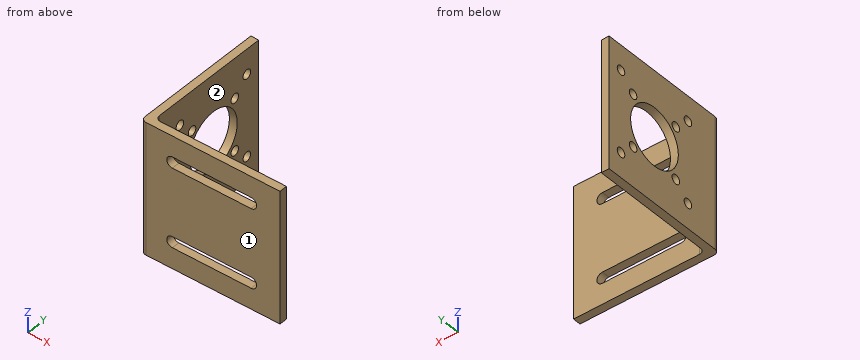
from build123d import *

# Parameters (mm, degrees)
SKETCH1_W           = 53
SKETCH1_H           = 50
BOSS_EXTRUDE1_DEPTH = 3
SKETCH2_W           = 3
SKETCH2_H           = 50
BOSS_EXTRUDE2_DEPTH = 48
CUT_EXTRUDE1_DEPTH  = 4
FILLET1_R           = 2
SKETCH4_R           = 1.75
SKETCH4_R_2         = 11.05
CUT_EXTRUDE2_DEPTH  = 4


with BuildPart() as part:
    # Sketch1 → Boss-Extrude1 (new body)
    with BuildSketch(Plane(origin=(0, 0, 0), x_dir=(1, 0, 0), z_dir=(0, 1, 0))):
        with Locations((26.5, 25)):
            Rectangle(SKETCH1_W, SKETCH1_H)
    extrude(amount=BOSS_EXTRUDE1_DEPTH)

    # Sketch2 → Boss-Extrude2 (add)
    with BuildSketch(Plane(origin=(0, 3, 0), x_dir=(1, 0, 0), z_dir=(0, 1, 0))):
        with Locations((1.5, 25)):
            Rectangle(SKETCH2_W, SKETCH2_H)
    extrude(amount=BOSS_EXTRUDE2_DEPTH)

    # Sketch3 → Cut-Extrude1 (cut, through all)
    with BuildSketch(Plane(origin=(0, 3, 0), x_dir=(1, 0, 0), z_dir=(0, 1, 0))):
        with BuildLine():
            Line((12, 37.9), (42, 37.9))
            ThreePointArc((42, 37.9), (44.1, 40), (42, 42.1))
            Line((42, 42.1), (12, 42.1))
            ThreePointArc((12, 42.1), (9.9, 40), (12, 37.9))
        make_face()
        with BuildLine():
            ThreePointArc((42, 12.1), (44.1, 10), (42, 7.9))
            Line((42, 7.9), (12, 7.9))
            ThreePointArc((12, 7.9), (9.9, 10), (12, 12.1))
            Line((12, 12.1), (42, 12.1))
        make_face()
    extrude(amount=-CUT_EXTRUDE1_DEPTH, mode=Mode.SUBTRACT)

    # Fillet1
    fillet1_edges = [part.edges().sort_by_distance(p)[0] for p in [
        (3, 3, -25),
        (0, 0, -25),
    ]]
    fillet(fillet1_edges, radius=FILLET1_R)

    # Sketch4 → Cut-Extrude2 (cut, through all)
    with BuildSketch(Plane(origin=(3, 0, 0), x_dir=(0, 0, -1), z_dir=(1, 0, 0))):
        with Locations((9.5, 45.5)):
            Circle(SKETCH4_R)
        with Locations((15.101010153, 39.9)):
            Circle(SKETCH4_R)
        with Locations((25, 30)):
            Circle(SKETCH4_R_2)
        with Locations((15.101010153, 20.1)):
            Circle(SKETCH4_R)
        with Locations((9.5, 14.5)):
            Circle(SKETCH4_R)
        with Locations((34.898989847, 20.1)):
            Circle(SKETCH4_R)
        with Locations((40.5, 14.5)):
            Circle(SKETCH4_R)
        with Locations((34.898989847, 39.9)):
            Circle(SKETCH4_R)
        with Locations((40.5, 45.5)):
            Circle(SKETCH4_R)
    extrude(amount=-CUT_EXTRUDE2_DEPTH, mode=Mode.SUBTRACT)


solid = part.part
Can you work these out from the model? Positions are in its coordinate system, mm. Face numbers are marked on the shaded views. A direction names the side the tool comes from. Give positions to 0.01 mm unless a question says otherwise; leave off trailing zeros. Loops run counter-clockwise (first coordinate to the right, second up) from the corner with the lowest first, then second, coordinate; pieces in that order, holes last. Notation, with made-up numbers: (0, -35.75) -> (10, -35.75) arc R12 ccw to (10, -14.75) -> close; hole circle Ø4 at (-30, 37). An arc over 180 degrees is marked (long way). Write item = value, one per line.
1) Will these pins go through, and if not, where does the flat tip stop? pin 1 (1 mm diameter, centred on x = 43, z = -12, fed in from +Y); pin 2 (2 mm diameter, centred on y = 39.9, z = -15.1, fed in from +X); pin 3 (2 mm diameter, centred on y = 28.5, z = -12, fed in from +X).
Check result:
pin_1 = 3
pin_2 = through
pin_3 = 3
2) For the marked faces 1 and 2, which set-ups out of +Z, -Z, +X, -X, +Y, -Y let a thin tool reach every point of the face, with its end or its side?
Check result:
face_1 = +Z, -Z, +X, -X, -Y
face_2 = +Z, -Z, +X, +Y
3) Suppose I cut it at B-B on y = 45.5. Write out the boundary of the cut face in (x, z).
Check result:
outline = (0, -50) -> (3, -50) -> (3, -42.25) -> (0, -42.25) -> close; (0, -38.75) -> (3, -38.75) -> (3, -11.25) -> (0, -11.25) -> close; (0, -7.75) -> (3, -7.75) -> (3, 0) -> (0, 0) -> close
4) Suppose I cut it at A-A on x = 28.5. Write out the boundary of the cut face in (y, z).
Check result:
outline = (0, -50) -> (3, -50) -> (3, -42.1) -> (0, -42.1) -> close; (0, -37.9) -> (3, -37.9) -> (3, -12.1) -> (0, -12.1) -> close; (0, -7.9) -> (3, -7.9) -> (3, 0) -> (0, 0) -> close
5) Suppose I cut it at C-C on z = -40. Write out the boundary of the cut face in (x, y), then the cut area to 3 significant figures.
Check result:
outline = (0, 2) arc R2 ccw to (2, 0) -> (9.9, 0) -> (9.9, 3) -> (5, 3) arc R2 cw to (3, 5) -> (3, 12.82) -> (0, 12.82) -> close; (0, 16.18) -> (3, 16.18) -> (3, 43.82) -> (0, 43.82) -> close; (0, 47.18) -> (3, 47.18) -> (3, 51) -> (0, 51) -> close; (44.1, 0) -> (53, 0) -> (53, 3) -> (44.1, 3) -> close
area = 180 mm2
6) I need wall thicknesses on L1, parallel to Y at x = 46, z = -17; L2, parallel to Y at x = 1.65, z = -40.5. Which ranges of each line are inside material? Lowest first, please. Write a range as from..to.
Check result:
L1 = 0..3
L2 = 0.03..12.75, 16.25..43.75, 47.25..51
7) Suppose I cut it at D-D on y = 30. Write out the boundary of the cut face in (x, z).
Check result:
outline = (0, -50) -> (3, -50) -> (3, -36.05) -> (0, -36.05) -> close; (0, -13.95) -> (3, -13.95) -> (3, 0) -> (0, 0) -> close
